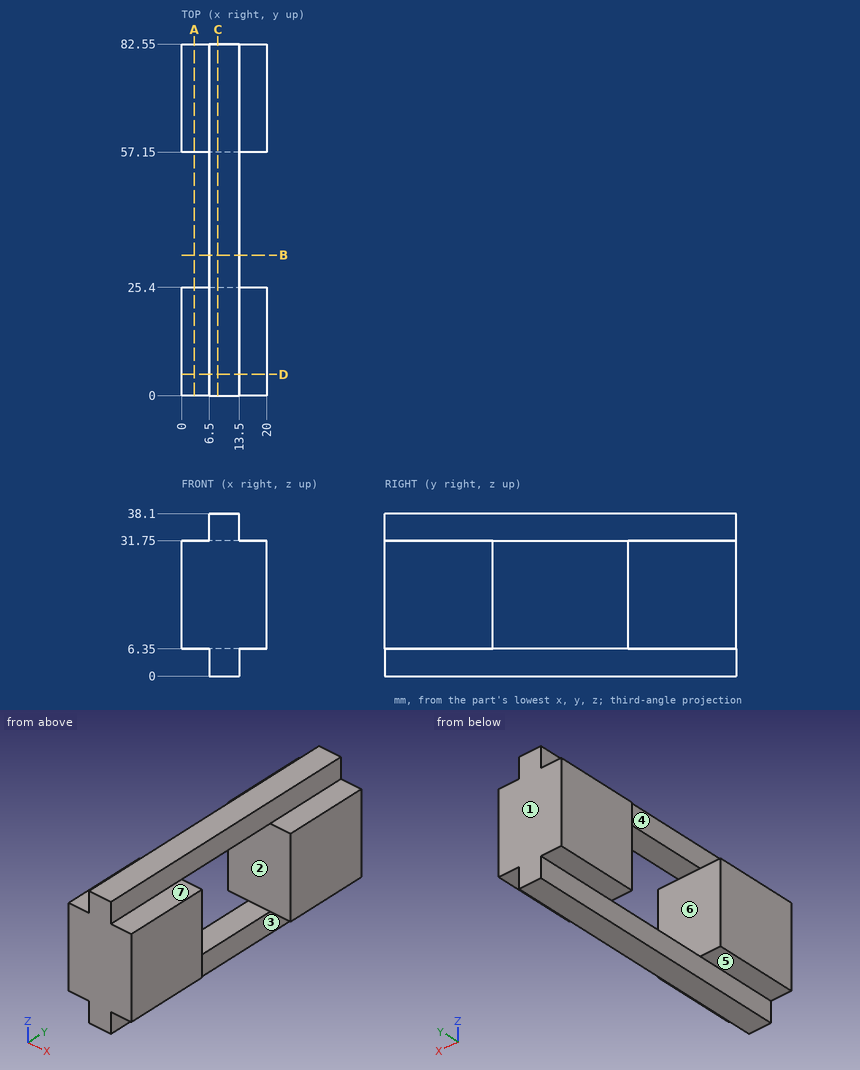
Answer from the drawing. Dimensions are ordinates in mm from the lowest x, y and z of the part. A direction names the side the tool comes from. Round coordinates to 2 decimals unless told otherwise and drop trailing zeros. Write each loop counter-clockwise with the first axis right and the second up, starting at its lowest first coordinate (ties: lowest second). Pieces come first, ordered by that corner, then holes. Notation, with made-up numbers: M 6.25,2 L 26.25,2 A28 ccw 26.25,22 Z; hole C 22.5,11.25 d5. An arc over 180 degrees is marked long. Write each question's results on one line, items separated by ' | '. Start each with the question number.
Item 1: For the marked faces 4, 5, 6 and 7, determine the directions among +Z, -Z, +X, -X, +Y, -Y from which every point of the face is accessible in a straight line to the end or side of a thin tool.
Item 2: A cutting plane is placed at C-C on x = 8.5. Write down the section's boundary in (y, z).
Item 3: For a pull along Y with two mould halves and no side action, classify the marked faces 1, 2 and 3 as pulls with the +Y half, pulls with the -Y half, needs draft (parallel to the pull), parting line crosses it, or undercut.
Item 4: A cutting plane is placed at A-A on x = 3. Write down the section's boundary in (y, z).
Item 5: Flat-ended cylindrical pins translate along their axes: pin 1 Ø3 at (y, z) = (53, 34) entering from +X; pin 2 Ø7 at (x, y) = (18.5, 75.5) entering from +Z; pin 3 Ø3.5 at (x, y) = (4, 73) entering from -Z; pin 4 Ø1.5 at (x, y) = (5, 28) entering from -Z. Find the tip coordinate at first contact, or state that the pin passes through.
Item 6: A cutting plane is placed at D-D on y = 5. Write down the section's boundary in (x, z).
Item 7: A cutting plane is placed at B-B on y = 33. Write down the section's boundary in (x, z), and give its area (3 significant figures).
Item 8: Straight lines are drawn through the part: L1, parallel to Y at x = 10.5, z = 7.5; L2, parallel to Z at x = 10, y = 55.5; L3, parallel to X at y = 72, z = 2. For each, find the intervals that lie inside material, in ascending order. Write a range as [from, to].
Check sheet entries:
1) face 4: +Z, -X, +Y, -Y | face 5: -Z, -X, +Y, -Y | face 6: +X, -X | face 7: +Z, +X, +Y, -Y
2) outline: M 0,0 L 82.55,0 L 82.55,38.1 L 0,38.1 Z; hole M 25.4,6.35 L 57.15,6.35 L 57.15,31.75 L 25.4,31.75 Z
3) face 1: pulls with the +Y half | face 2: undercut | face 3: needs draft
4) outline: M 0,6.35 L 25.4,6.35 L 25.4,31.75 L 0,31.75 Z; M 57.15,6.35 L 82.55,6.35 L 82.55,31.75 L 57.15,31.75 Z
5) pin 1: x = 13.5 | pin 2: z = 31.75 | pin 3: z = 6.35 | pin 4: through
6) outline: M 0,6.35 L 6.5,6.35 L 6.5,0 L 13.5,0 L 13.5,6.35 L 20,6.35 L 20,31.75 L 13.5,31.75 L 13.5,38.1 L 6.5,38.1 L 6.5,31.75 L 0,31.75 Z
7) outline: M 6.5,0 L 13.5,0 L 13.5,6.35 L 6.5,6.35 Z; M 6.5,31.75 L 13.5,31.75 L 13.5,38.1 L 6.5,38.1 Z | area: 88.9 mm²
8) L1: [0, 25.4], [57.15, 82.55] | L2: [0, 6.35], [31.75, 38.1] | L3: [6.5, 13.5]
